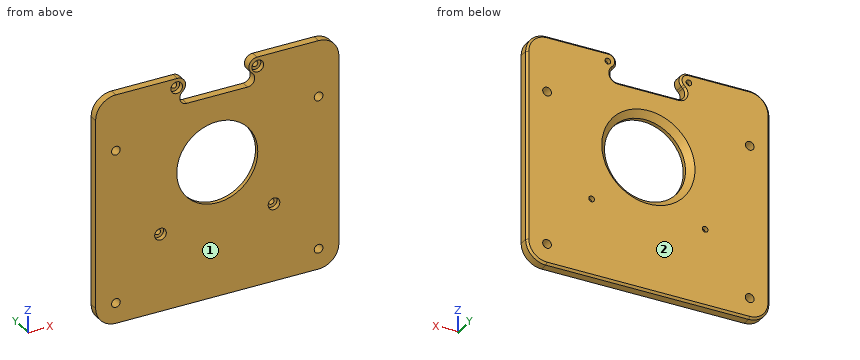
from build123d import *

# Parameters (mm, degrees)
SKETCH2_W           = 120
SKETCH2_H           = 112.5
BOSS_EXTRUDE2_DEPTH = 5
CUT_EXTRUDE7_DEPTH  = 6
FILLET5_R           = 10
SKETCH10_R          = 20
CUT_EXTRUDE9_DEPTH  = 6
CHAMFER3_SIZE       = 3
FILLET6_R           = 4
CHAMFER4_SIZE       = 1
SKETCH11_R          = 2.15
CUT_EXTRUDE10_DEPTH = 6
SKETCH1_R           = 1.4
CUT_EXTRUDE13_DEPTH = 5
SKETCH13_R          = 2.875
CUT_EXTRUDE12_DEPTH = 2.5


with BuildPart() as part:
    # Sketch2 → Boss-Extrude2 (new body)
    with BuildSketch(Plane(origin=(0, 0, 0), x_dir=(1, 0, 0), z_dir=(0, 1, 0))):
        with Locations((0, 9.75)):
            Rectangle(SKETCH2_W, SKETCH2_H)
    extrude(amount=BOSS_EXTRUDE2_DEPTH)

    # Sketch9 → Cut-Extrude7 (cut, through all)
    with BuildSketch(Plane(origin=(0, 5, 0), x_dir=(1, 0, 0), z_dir=(0, 1, 0))):
        with BuildLine():
            ThreePointArc((-15, -33), (-18.232806931, -35.158747099), (-17.477720957, -38.972023232))
            Line((-17.477720957, -38.972023232), (-10.196302495, -46.5))
            Line((-10.196302495, -46.5), (10.196302495, -46.5))
            Line((10.196302495, -46.5), (17.477720957, -38.972023232))
            ThreePointArc((17.477720957, -38.972023232), (18.232806931, -35.158747099), (15, -33))
            Line((15, -33), (-15, -33))
        make_face()
    extrude(amount=-CUT_EXTRUDE7_DEPTH, mode=Mode.SUBTRACT)

    # Fillet5
    fillet5_edges = [part.edges().sort_by_distance(p)[0] for p in [
        (-60, 2.5, -66),
        (60, 2.5, -66),
        (60, 2.5, 46.5),
        (-60, 2.5, 46.5),
    ]]
    fillet(fillet5_edges, radius=FILLET5_R)

    # Sketch10 → Cut-Extrude9 (cut, through all)
    with BuildSketch(Plane(origin=(0, 0, 0), x_dir=(1, 0, 0), z_dir=(0, 1, 0))):
        Circle(SKETCH10_R)
    extrude(amount=CUT_EXTRUDE9_DEPTH, mode=Mode.SUBTRACT)

    # Chamfer3
    chamfer3_edges = [part.edges().sort_by_distance(p)[0] for p in [
        (-20, 5, 0),
    ]]
    chamfer(chamfer3_edges, length=CHAMFER3_SIZE)

    # Fillet6
    fillet6_edges = [part.edges().sort_by_distance(p)[0] for p in [
        (10.196302495, 2.5, 46.5),
        (-10.196302495, 2.5, 46.5),
    ]]
    fillet(fillet6_edges, radius=FILLET6_R)

    # Chamfer4
    chamfer4_edges = [part.edges().sort_by_distance(p)[0] for p in [
        (18.232806931, 5, 35.158747099),
        (17.116441895, 5, 39.345535673),
        (-18.232806931, 5, 35.158747099),
        (0, 5, 33),
        (-17.116441895, 5, 39.345535673),
        (-60, 5, -9.75),
        (0, 5, -66),
        (60, 5, -9.75),
        (-34.815140686, 5, 46.5),
        (-57.071067812, 5, 43.571067812),
        (57.071067812, 5, 43.571067812),
        (57.071067812, 5, -63.071067812),
        (-57.071067812, 5, -63.071067812),
        (34.815140686, 5, 46.5),
        (15.947632356, 5, 44.061440433),
        (-15.947632356, 5, 44.061440433),
    ]]
    chamfer(chamfer4_edges, length=CHAMFER4_SIZE)

    # Sketch11 → Cut-Extrude10 (cut, through all)
    with BuildSketch(Plane(origin=(0, 5, 0), x_dir=(1, 0, 0), z_dir=(0, 1, 0))):
        with Locations((-50, 56)):
            Circle(SKETCH11_R)
        with Locations((50, 56)):
            Circle(SKETCH11_R)
        with Locations((-50, -19)):
            Circle(SKETCH11_R)
        with Locations((50, -19)):
            Circle(SKETCH11_R)
    extrude(amount=-CUT_EXTRUDE10_DEPTH, mode=Mode.SUBTRACT)

    # Sketch1 → Cut-Extrude13 (cut)
    with BuildSketch(Plane(origin=(0, 0, 0), x_dir=(1, 0, 0), z_dir=(0, 1, 0))):
        with Locations((-20, -42)):
            Circle(SKETCH1_R)
        with Locations((20, -42)):
            Circle(SKETCH1_R)
        with Locations((28, 28)):
            Circle(SKETCH1_R)
        with Locations((-28, 28)):
            Circle(SKETCH1_R)
    extrude(amount=CUT_EXTRUDE13_DEPTH, mode=Mode.SUBTRACT)

    # Sketch13 → Cut-Extrude12 (cut)
    with BuildSketch(Plane.XZ):
        with Locations((-20, 42)):
            Circle(SKETCH13_R)
        with Locations((20, 42)):
            Circle(SKETCH13_R)
        with Locations((-28, -28)):
            Circle(SKETCH13_R)
        with Locations((28, -28)):
            Circle(SKETCH13_R)
    extrude(amount=-CUT_EXTRUDE12_DEPTH, mode=Mode.SUBTRACT)


solid = part.part
For this review, take the finished solid that the model builds, in its own axes (mm). Face numbers are marked on the shaded views. Give positions to 0.01 mm unless a question says otherwise; leave off trailing zeros. Write each loop counter-clockwise with the first axis right and the second up, starting at its lowest first coordinate (ties: lowest second). Pieces come first, ordered by that corner, then holes. Notation, with made-up numbers: (42.25, -34) -> (93.25, -34) arc R37 ccw to (93.25, 3) -> close; hole circle Ø7 at (70.5, 58). An arc over 180 degrees is marked (long way). Use CSV: the item, a comma, the result in double quotes.
Q1. Mouldability with a two-part tool opening along Y and no side actions: class the marked faces 1 and 2 as pulls with the +Y half, pulls with the -Y half, needs draft (parallel to the pull), parting line crosses it, or undercut.
Conclusion:
face 1,"pulls with the -Y half"
face 2,"pulls with the +Y half"
Q2. Take a section at A-A, the plane x = 0. Write out the cut boundary in (y, z), then the cut area to 3 significant figures.
Conclusion:
outline,"(0, -66) -> (4, -66) -> (5, -65) -> (5, -23) -> (2, -20) -> (0, -20) -> close; (0, 20) -> (2, 20) -> (5, 23) -> (5, 32) -> (4, 33) -> (0, 33) -> close"
area,"285 mm2"
Q3. Take a section at B-B, the plane z = 0. Write out the cut boundary in (x, y), then the cut area to 3 significant figures.
Conclusion:
outline,"(-60, 0) -> (-20, 0) -> (-20, 2) -> (-23, 5) -> (-59, 5) -> (-60, 4) -> close; (20, 0) -> (60, 0) -> (60, 4) -> (59, 5) -> (23, 5) -> (20, 2) -> close"
area,"390 mm2"
Q4. For P1, Ø6, axis at x = -18, z = -7, coming from the +Y side; P2, Ø3, axis at x = -19.5, z = 41, coming from the -Y side; P3, Ø1.5, axis at x = 19.5, z = 10.5, coming from the +Y side; P4, Ø2.5, axis at x = -50, z = 19, coming from the -Y side, all flat-tipped, find the tip position at first contact; note any pin that passes through.
Conclusion:
P1,"y = 4.31"
P2,"y = 2.5"
P3,"y = 4.9"
P4,"through"
Q5. Take a section at C-C, the plane y = 0.8. State how many separate pieces and enclosed holes the cut face has, then the cut area to 3 significant figures.
Conclusion:
separate pieces,"1"
enclosed holes,"9"
area,"11,500 mm2"
Q6. To check wall thickness, follow probe 1 along Z at (x, y) = (-50, 1.4); probe 2 along Z at (x, y) = (-28, 1.1) (3 decimals); probe 3 along Z at (x, y) = (11.5, 2.7). State the ranges of each line that lie inside material, in increasing order. Write a range as [from, to].
Conclusion:
probe 1,"[-66, -58.15], [-53.85, 16.85], [21.15, 46.5]"
probe 2,"[-66, -30.875], [-25.125, 46.5]"
probe 3,"[-66, -17.21], [17.21, 33]"
Q7. Take a section at D-D, the plane z = -28. Write out the cut boundary in (x, y) (3 decimals).
Conclusion:
outline,"(-60, 0) -> (-30.875, 0) -> (-30.875, 2.5) -> (-29.4, 2.5) -> (-29.4, 5) -> (-59, 5) -> (-60, 4) -> close; (-26.6, 2.5) -> (-25.125, 2.5) -> (-25.125, 0) -> (25.125, 0) -> (25.125, 2.5) -> (26.6, 2.5) -> (26.6, 5) -> (-26.6, 5) -> close; (29.4, 2.5) -> (30.875, 2.5) -> (30.875, 0) -> (60, 0) -> (60, 4) -> (59, 5) -> (29.4, 5) -> close"
